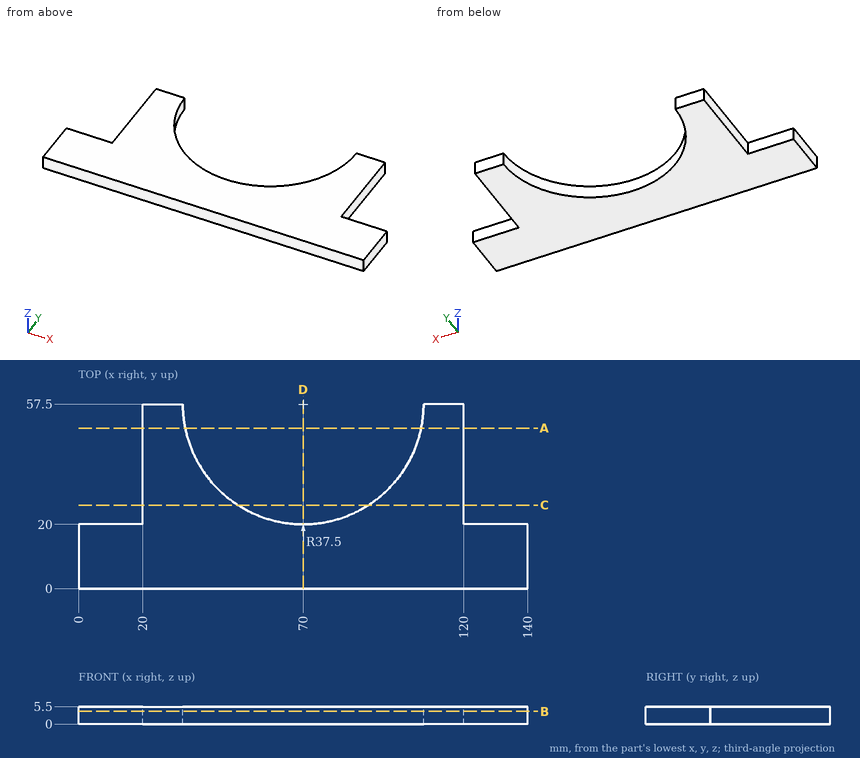
Could you check a few things on this drawing? It's one solid part, dimensions in mm from its lowest x, y, z. Coordinates: 2 decimals unless noted, no trailing zeros. Write each loop counter-clockwise with the first axis right and the second up, starting at its lowest first coordinate (ties: lowest second). Pieces come first, ordered by that corner, then holes. Notation, with made-up numbers: (66, 32) - (79, 32) arc R12 cw to (79, 51) - close; hole circle Ø11 at (-30, 84.5). An arc over 180 degrees is marked (long way). Put each result on its own line as item: value. Start each with the question number.
Q1. I want a section at A-A on y = 50. Write out the boundary of the cut face in (x, z), plus the area to 3 significant figures.
Q2. Please list where these lines run through material, in increasing order: L1, parallel to Y at x = 132, z = 3.75; L2, parallel to X at y = 34, z = 0.9; L3, parallel to X at y = 33, z = 2.1.
Q3. I want a section at D-D on x = 70. Write out the boundary of the cut face in (y, z).
Q4. I'm going to push a flat-ended pin straight in: P1, Ø3, axis at x = 8, z = 3, coming from the +Y side. Where does the tip first touch, or does it pass through?
Q5. I want a section at C-C on y = 26. Write out the boundary of the cut face in (x, z), plus the area to 3 significant figures.
Q6. I want a section at B-B on z = 4. Write out the boundary of the cut face in (x, y), plus the area to 3 significant figures.
Checks:
1. outline: (20, 0) - (33.26, 0) - (33.26, 5.5) - (20, 5.5) - close; (106.74, 0) - (120, 0) - (120, 5.5) - (106.74, 5.5) - close
1. area: 146 mm²
2. L1: 0 to 20
2. L2: 20 to 40.78, 99.22 to 120
2. L3: 20 to 41.61, 98.39 to 120
3. outline: (0, 0) - (20, 0) - (20, 5.5) - (0, 5.5) - close
4. P1: y = 20
5. outline: (20, 0) - (49.65, 0) - (49.65, 5.5) - (20, 5.5) - close; (90.35, 0) - (120, 0) - (120, 5.5) - (90.35, 5.5) - close
5. area: 326 mm²
6. outline: (0, 0) - (140, 0) - (140, 20) - (120, 20) - (120, 57.5) - (107.5, 57.5) arc R37.5 cw to (32.5, 57.5) - (20, 57.5) - (20, 20) - (0, 20) - close
6. area: 4,340 mm²
